Geometry check sheet. Reference: drawing and pictorial views, mm from the part's lowest x, y, z. Round coordinates to 2 decimals unless told otherwise and drop trailing zeros. Order: outer loops, then holes, each group sorted by start corner. A loop starts at its lowest first (then second) coordinate and runs counter-clockwise, first axis right, second up.
(1) Depth check by flat-ended pin: pin 1 (5 mm diameter, centred on x = 57.15, y = 19.05, fed in from -Z). Enter the tip coordinate at first touch or a pass-through.
(2) Sectioned sample at A-A, the plane y = 57.15. Enter the section's corners in (x, z), and give its area (3 significant figures).
(3) Sectioned sample at C-C, the plane x = 133.35. Enter the section's corners in (y, z), and give its area (3 significant figures).
(4) Thickness scan on probe 1 along Y at (x, z) = (57.15, 5); probe 2 along X at (y, z) = (60, 2.25). Record the ranges inside material, lowest first.
(5) Sectioned sample at B-B, the plane z = 1.75. Count the separate pieces of the cut face and the enclosed holes in it, and give its area (3 significant figures).
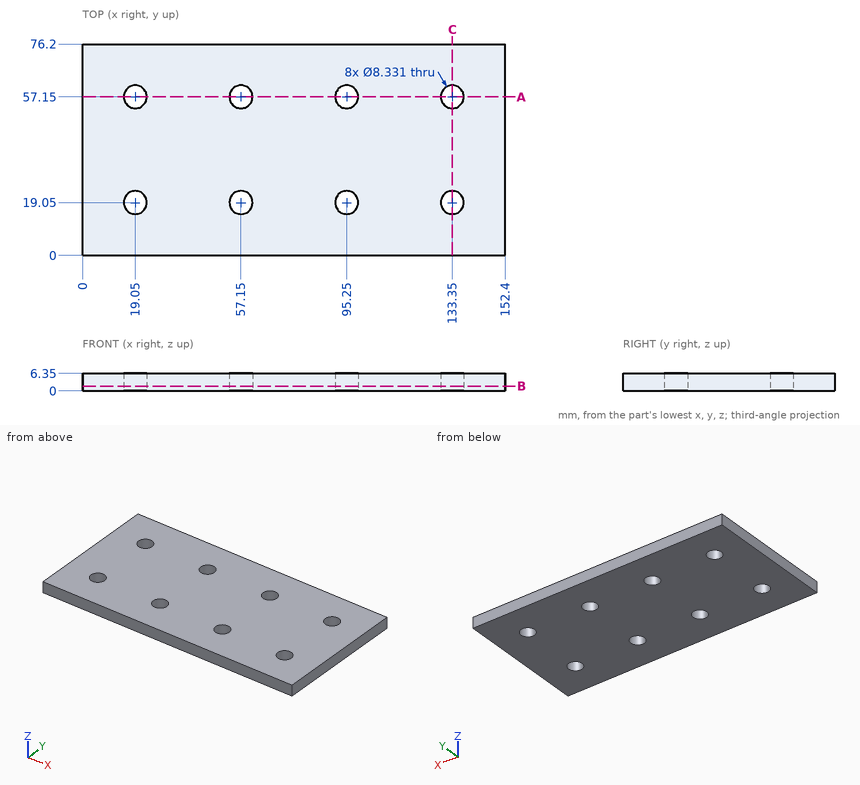
Derived:
1. pin 1: passes through
2. outline: (0, 0) - (14.88, 0) - (14.88, 6.35) - (0, 6.35) - close; (23.22, 0) - (52.98, 0) - (52.98, 6.35) - (23.22, 6.35) - close; (61.32, 0) - (91.08, 0) - (91.08, 6.35) - (61.32, 6.35) - close; (99.42, 0) - (129.18, 0) - (129.18, 6.35) - (99.42, 6.35) - close; (137.52, 0) - (152.4, 0) - (152.4, 6.35) - (137.52, 6.35) - close
2. area: 756 mm2
3. outline: (0, 0) - (14.88, 0) - (14.88, 6.35) - (0, 6.35) - close; (23.22, 0) - (52.98, 0) - (52.98, 6.35) - (23.22, 6.35) - close; (61.32, 0) - (76.2, 0) - (76.2, 6.35) - (61.32, 6.35) - close
3. area: 378 mm2
4. probe 1: y = 0 to 14.88, 23.22 to 52.98, 61.32 to 76.2
4. probe 2: x = 0 to 16.01, 22.09 to 54.11, 60.19 to 92.21, 98.29 to 130.31, 136.39 to 152.4
5. separate pieces: 1
5. enclosed holes: 8
5. area: 11,200 mm2
